Here's the drawing with two shaded views (mm, measured from the low corner). I have some questions. A direction names the side the tool comes from. Coordinates: 2 decimals unless noted, no trailing zeros. Write each loop counter-clockwise with the first axis right and the second up, starting at its lowest first coordinate (ties: lowest second). Pieces come first, ordered by that corner, then holes.
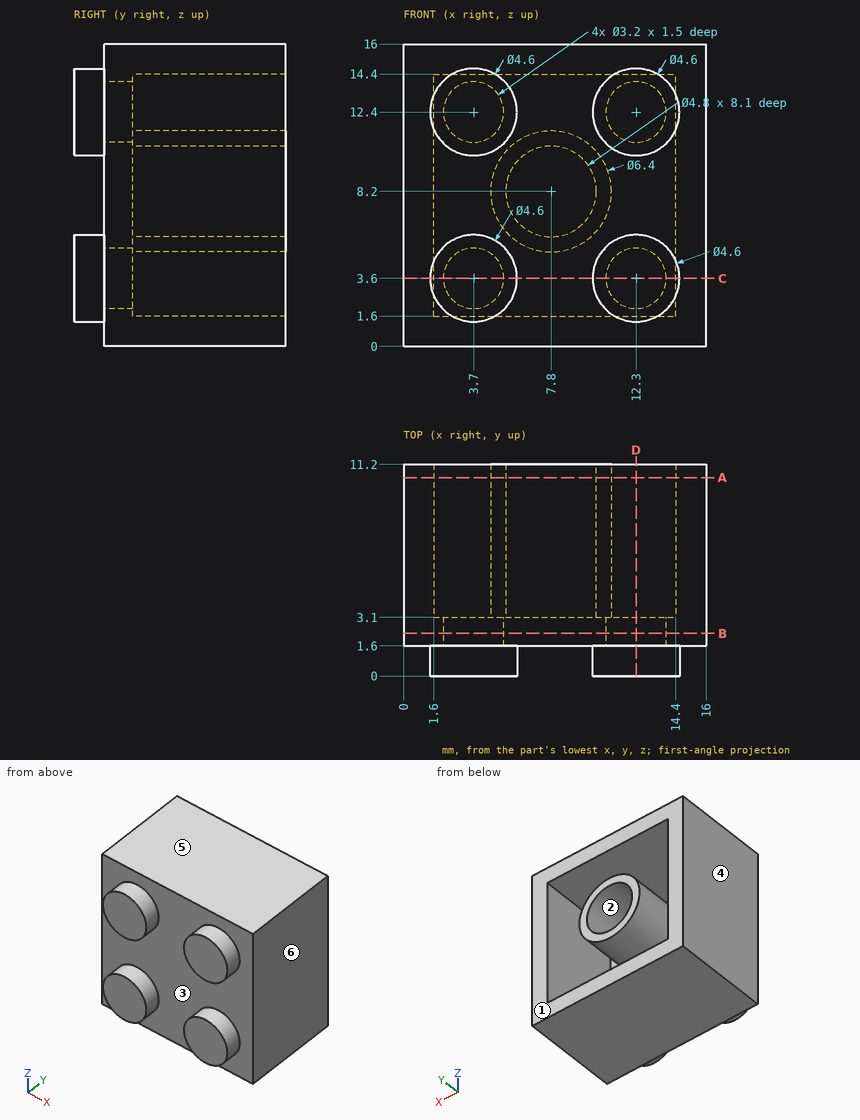
Item 1: Which directions (+Z, -Z, +X, -X, +Y, -Y) give clear straight access to the entire face, cutting with the end or side of a thin tool? Please do the marked faces 1 and 2.
Item 2: I want a section at D-D, the plane x = 12.3. List the corners of the cut face in (y, z) for me.
Item 3: I want a section at B-B, the plane y = 2.25. List the corners of the cut face in (x, z) for me, then the cut area to 3 significant figures.
Item 4: If we mould it in two halves opening along X, with no side actions, what happens to the marked faces 3, 4, 5 and 6? For each: released by +X, released by -X, zero draft, split by the parting line, or undercut.
Item 5: If I drill on line 1 along Z through (x, y) = (12.3, 2.35); line 2 along X through (y, z) = (9.25, 6.5); line 3 along X through (y, z) = (2.5, 13.75), over which ranges is the centre line in solid material (lowest first)?
Item 6: Will these pins go through, and if not, where does the flat tip stop? pin 1 Ø1.4 at (x, z) = (7, 9) entering from +Y; pin 2 Ø1 at (x, z) = (11.5, 13) entering from +Y; pin 3 Ø4.5 at (x, z) = (7.8, 8.2) entering from -Y.
Item 7: I want a section at A-A, the plane y = 10.5. List the corners of the cut face in (x, z) for me.
Item 8: I want a section at C-C, the plane z = 3.6. List the corners of the cut face in (x, y) for me.
Taken from the geometry:
1. face 1: +Z, -Z, +X, -X, +Y
1. face 2: +Y
2. outline: (0, 1.3) - (1.6, 1.3) - (1.6, 0) - (11.2, 0) - (11.2, 1.6) - (3.1, 1.6) - (3.1, 2) - (1.6, 2) - (1.6, 5.2) - (3.1, 5.2) - (3.1, 10.8) - (1.6, 10.8) - (1.6, 14) - (3.1, 14) - (3.1, 14.4) - (11.2, 14.4) - (11.2, 16) - (1.6, 16) - (1.6, 14.7) - (0, 14.7) - (0, 10.1) - (1.6, 10.1) - (1.6, 5.9) - (0, 5.9) - close
3. outline: (0, 0) - (16, 0) - (16, 16) - (0, 16) - close; hole circle Ø3.2 at (3.7, 3.6); hole circle Ø3.2 at (3.7, 12.4); hole circle Ø3.2 at (12.3, 3.6); hole circle Ø3.2 at (12.3, 12.4)
3. area: 224 mm2
4. face 3: undercut
4. face 4: released by -X
4. face 5: zero draft
4. face 6: released by +X
5. line 1: z = 0 to 2, 5.2 to 10.8, 14 to 16
5. line 2: x = 0 to 1.6, 5.09 to 6.11, 9.49 to 10.51, 14.4 to 16
5. line 3: x = 0 to 2.84, 4.56 to 11.44, 13.16 to 16
6. pin 1: stops at y = 3.1
6. pin 2: stops at y = 1.6
6. pin 3: stops at y = 1.6
7. outline: (0, 0) - (16, 0) - (16, 16) - (0, 16) - close; circle Ø6.4 at (7.8, 8.2); hole (1.6, 1.6) - (14.4, 1.6) - (14.4, 14.4) - (1.6, 14.4) - close; hole circle Ø4.8 at (7.8, 8.2)
8. outline: (0, 1.6) - (1.4, 1.6) - (1.4, 0) - (6, 0) - (6, 1.6) - (10, 1.6) - (10, 0) - (14.6, 0) - (14.6, 1.6) - (16, 1.6) - (16, 11.2) - (14.4, 11.2) - (14.4, 3.1) - (13.9, 3.1) - (13.9, 1.6) - (10.7, 1.6) - (10.7, 3.1) - (5.3, 3.1) - (5.3, 1.6) - (2.1, 1.6) - (2.1, 3.1) - (1.6, 3.1) - (1.6, 11.2) - (0, 11.2) - close
